Job drawing, mm, ordinate dimensions from the low corner. One solid piece. Round coordinates to 2 decimals unless told otherwise and drop trailing zeros. Loops run counter-clockwise (first coordinate to the right, second up) from the corner with the lowest first, then second, coordinate; pieces in that order, holes last.
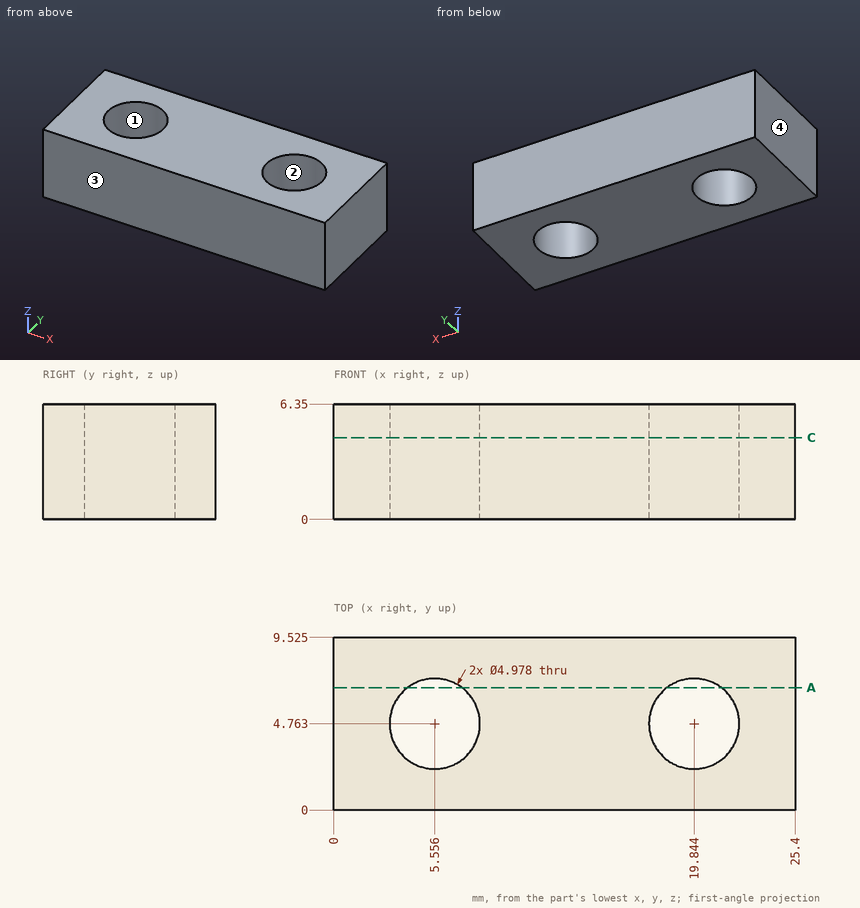
1) Slice it at C-C, the plane z = 4.5. Give the cut face in (x, y) (1 decimal).
Values:
outline: (0, 0) - (25.4, 0) - (25.4, 9.5) - (0, 9.5) - close; hole circle Ø5 at (5.6, 4.8); hole circle Ø5 at (19.8, 4.8)
2) Wall check: line 1 along X through (y, z) = (4.75, 6) (1 decimal); line 2 along X through (y, z) = (6.5, 1) (1 decimal); line 3 along Y through (x, z) = (21.75, 6.25) (1 decimal). Give the ranges that are in metal, low to high.
Values:
line 1: x = 0 to 3.1, 8 to 17.4, 22.3 to 25.4
line 2: x = 0 to 3.8, 7.3 to 18.1, 21.6 to 25.4
line 3: y = 0 to 3.2, 6.4 to 9.5
3) Mould opens along Y. For the marked faces 1, 2, 3 and 4 say: released by +Y, released by -Y, zero draft, split by the parting line, or undercut.
Values:
face 1: undercut
face 2: undercut
face 3: released by -Y
face 4: zero draft
4) Slice it at A-A, the plane y = 6.75. Give the number of separate pieces and of enclosed holes in the cut face, then the cut area to 3 significant figures.
Values:
separate pieces: 3
enclosed holes: 0
area: 123 mm2
